Source: CAD feature listing. Evaluate the final solid. Frame: model axes, mm. Give positions to 0.01 mm unless a question says otherwise; leave off trailing zeros. Write each loop counter-clockwise with the first axis right and the second up, starting at its lowest first coordinate (ties: lowest second). Pieces come first, ordered by that corner, then holes. Notation, with made-up numbers: M 7.5,68 L 25.5,68 A18 ccw 25.5,75 Z; hole C 7.25,-27.5 d6. An arc over 180 degrees is marked long. Return JSON: item names as keys, results as strings.
```python
from build123d import *
from build123d import SkipClean  # not in build123d's __all__

# Parameters (mm, degrees)
F0_W           = 93
F0_H           = 15.05
F1_DEPTH       = 1.5
F2_W           = 15.05
F2_H           = 13
F3_DEPTH       = 1.5
F4_R           = 2
F6_DEPTH       = 1.5
F7_R           = 2
F9_DEPTH       = 93
F11_DEPTH      = 10.5
F13_DEPTH      = 90
F15_W          = 8
F15_H          = 8.5
F16_DEPTH      = 2.5
F16_DEPTH_BACK = 2.5


# Not quite as in the source:
# - after a boolean that leaves OpenCascade's solid faulty, fix() repairs it
# - a feature names something its author has since deleted; it is built from what else it names


with BuildPart() as f1:
    # F0 (on Top) → F1 (new body)
    with BuildSketch(Plane.XY):
        with Locations((0, -8.8193283182)):
            Rectangle(F0_W, F0_H)
    extrude(amount=F1_DEPTH)

    # F2 (on face) → F3 (join)
    with BuildSketch(Plane(origin=(-46.5, 0, 0), x_dir=(0, -1, 0), z_dir=(-1, 0, 0))):
        with Locations((8.8193283182, 8)):
            Rectangle(F2_W, F2_H)
    extrude(amount=-F3_DEPTH)

    # F4
    f4_edges = [f1.edges().sort_by_distance(p)[0] for p in [
        (-46.5, -8.819328, 0),
    ]]
    fillet(f4_edges, radius=F4_R)

    # F5 (on face) → F6 (join)
    with BuildSketch(Plane.YZ.offset(46.5)):
        with BuildLine():
            Line((-16.3443283182, 10.475), (-16.3443283182, 0))
            Line((-16.3443283182, 0), (-1.2943283182, 0))
            Line((-1.2943283182, 0), (-1.2943283182, 10.475))
            ThreePointArc((-1.2943283182, 10.475), (-8.8193283182, 2.95), (-16.3443283182, 10.475))
        make_face()
        with BuildLine():
            ThreePointArc((-1.2943283182, 10.475), (-8.8193283182, 18), (-16.3443283182, 10.475))
            Line((-16.3443283182, 10.475), (-1.2943283182, 10.475))
        make_face()
        with BuildLine():
            Line((-1.2943283182, 10.475), (-16.3443283182, 10.475))
            ThreePointArc((-16.3443283182, 10.475), (-8.8193283182, 2.95), (-1.2943283182, 10.475))
        make_face()
    extrude(amount=-F6_DEPTH)

    # F7
    f7_edges = [f1.edges().sort_by_distance(p)[0] for p in [
        (46.5, -8.819328, 0),
    ]]
    fillet(f7_edges, radius=F7_R)

    # F8 (on face) → F9 (join)
    with BuildSketch(Plane.YZ.offset(46.5)):
        with BuildLine():
            ThreePointArc((-7.3193283182, 10.475), (-8.8193283182, 11.975), (-10.3193283182, 10.475))
            Line((-10.3193283182, 10.475), (-7.3193283182, 10.475))
        make_face()
        with BuildLine():
            Line((-7.3193283182, 10.475), (-10.3193283182, 10.475))
            ThreePointArc((-10.3193283182, 10.475), (-8.8193283182, 8.975), (-7.3193283182, 10.475))
        make_face()
    extrude(amount=-F9_DEPTH)

    # F10 (on face) → F11 (join)
    with BuildSketch(Plane.YZ.offset(46.5)):
        with BuildLine():
            ThreePointArc((-1.2943283182, 10.475), (-8.8193283182, 18), (-16.3443283182, 10.475))
            Line((-16.3443283182, 10.475), (-1.2943283182, 10.475))
        make_face()
        with BuildLine():
            Line((-1.2943283182, 10.475), (-16.3443283182, 10.475))
            ThreePointArc((-16.3443283182, 10.475), (-8.8193283182, 2.95), (-1.2943283182, 10.475))
        make_face()
    with SkipClean():  # cleaning this boolean's faces spoils the solid; the shape is the same uncleaned
        extrude(amount=F11_DEPTH)

    # F12 (on face) → F13 (join, through all)
    with BuildSketch(Plane.YZ.offset(-45)):
        with BuildLine():
            ThreePointArc((-12.3893283182, 6.5), (-13.8443283182, 7.955), (-15.2993283182, 6.5))
            Line((-15.2993283182, 6.5), (-13.8443283182, 6.5))
            Line((-13.8443283182, 6.5), (-12.3893283182, 6.5))
        make_face()
        with BuildLine():
            Line((-13.8443283182, 6.5), (-15.2993283182, 6.5))
            ThreePointArc((-15.2993283182, 6.5), (-13.8443283182, 5.045), (-12.3893283182, 6.5))
            Line((-12.3893283182, 6.5), (-13.8443283182, 6.5))
        make_face()
        with BuildLine():
            ThreePointArc((-5.2493283182, 6.5), (-3.7943283182, 5.045), (-2.3393283182, 6.5))
            Line((-2.3393283182, 6.5), (-3.7943283182, 6.5))
            Line((-3.7943283182, 6.5), (-5.2493283182, 6.5))
        make_face()
        with BuildLine():
            Line((-3.7943283182, 6.5), (-2.3393283182, 6.5))
            ThreePointArc((-2.3393283182, 6.5), (-3.7943283182, 7.955), (-5.2493283182, 6.5))
            Line((-5.2493283182, 6.5), (-3.7943283182, 6.5))
        make_face()
    extrude(amount=F13_DEPTH)

    add(f1.part.fix(), mode=Mode.REPLACE)

    # F15 (on offset) → F16 (join, two sides)
    with BuildSketch(Plane(origin=(0, -1.2943283182, 0), x_dir=(-1, 0, 0), z_dir=(0, 1, 0))) as f16_sk:
        with Locations((-52.5, 10.2375)):
            Rectangle(F15_W, F15_H)
    extrude(amount=F16_DEPTH)
    extrude(f16_sk.sketch, amount=-F16_DEPTH_BACK)


solid = f1.part
```
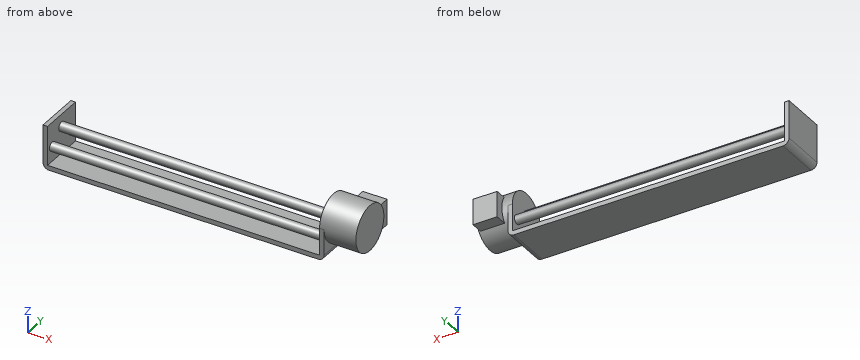
1) Line query: line 1 (X direction, y = -7.5, z = 13); line 2 (Z direction, x = -30.5, y = -4); line 3 (Y direction, x = 3, z = 6.25). Output: solid intervals per line, ascending. Write a range as [from, to].
Numbers:
{"line 1": "x = [-46.5, -45], [45, 57]", "line 2": "z = [0, 1.5], [5.06, 7.94]", "line 3": "y = [-15.28, -12.41], [-5.23, -2.36]"}
2) Cut plane C-C, the plane y = -6.25. Return the cut outline in (x, z), then the cut area to 3 significant figures.
Numbers:
{"outline": "M -46.5,2 A2 ccw -44.5,0 L 44.5,0 A2 ccw 46.5,2 L 46.5,3.4 L 57,3.4 L 57,17.55 L 45,17.55 L 45,1.5 L -45,1.5 L -45,14.5 L -46.5,14.5 Z", "area": "330 mm²"}
3) Cut plane D-D, the plane z = 16.75. Return the cut outline in (x, y), then the cut area to 3 significant figures.
Numbers:
{"outline": "M 45,-12.97 L 57,-12.97 L 57,-4.67 L 45,-4.67 Z", "area": "99.7 mm²"}
4) Contact query for flat-ended pins moving along their axis: pin 1 Ø6 at (x, z) = (-32.5, 2.5) entering from +Y; pin 2 Ø1.6 at (x, y) = (-46, -7) entering from +Z; pin 3 Ø2 at (x, y) = (52.5, 0) entering from -Z. Output: stop coordinate, or through.
Numbers:
{"pin 1": "stops at y = -1.29", "pin 2": "stops at z = 14.5", "pin 3": "stops at z = 5.99"}
5) Cut plane A-A, the plane x = -37.5. Return the cut outline in (y, z) (3 decimals).
Numbers:
{"outline": "M -16.344,0 L -1.294,0 L -1.294,1.5 L -16.344,1.5 Z; C -13.844,6.5 d2.91; C -8.819,10.475 d3; C -3.794,6.5 d2.91"}
6) Cut plane B-B, the plane y = -13.5. Return the cut outline in (x, z), then the cut area to 3 significant figures.
Numbers:
{"outline": "M -46.5,2 A2 ccw -44.5,0 L 44.5,0 A2 ccw 46.5,2 L 46.5,4.58 L 57,4.58 L 57,16.37 L 45,16.37 L 45,7.91 L -45,7.91 L -45,14.5 L -46.5,14.5 Z; hole M -45,1.5 L 45,1.5 L 45,5.09 L -45,5.09 Z", "area": "558 mm²"}
